The listing builds one solid part. Answer for the finished solid, in the listing's coordinates (mm). A direction names the side the tool comes from. Coordinates: 2 decimals unless noted, no trailing zeros. Order: outer loops, then holes, each group sorted by start corner. A loop starts at its lowest first (then second) coordinate and runs counter-clockwise, first axis right, second up. Notation, with made-up numbers: (89, 37.25) - (125, 37.25) arc R9 ccw to (125, 44.25) - close; hole circle Ø7 at (76, -5.75). An arc over 180 degrees is marked (long way). Use one line per item in the form item = value. Start each with the question number.
Item 1: Consider line 1 along Y through (x, z) = (142, 17.75); line 2 along X through (y, z) = (-28.5, 3); line 3 along X through (y, z) = (-70.5, 5.5). Determine where each line is inside the solid, lowest interval first. Write a range as [from, to].
Item 2: Section B-B, the plane x = 187.5 is taken. Write down the section's boundary in (y, z), and give its area (3 significant figures).
Item 3: The mould has two halves that part along Y. Classify faces 1 (the flat face through (355, 27, 8.89)), 2 (the flat face through (354, -2, 0)): released by +Y, released by -Y, zero draft, split by the parting line, or undercut.
Item 4: Each of these flat-tipped pins is pushed along its axis until it touches: pin 1 Ø1.9 at (y, z) = (31.5, 4) entering from -X; pin 2 Ø2 at (y, z) = (74.5, 12) entering from -X; pin 3 Ø23 at (x, y) = (342.5, -32.5) entering from +Z; pin 4 Ø1.9 at (y, z) = (28.5, 2) entering from +X. Where does it stop, or does it pass through?
Item 5: A tool of negligible diameter and unlimited length cuts with its end or side. For faces 3 (the flat face through (355, 88, 8.89)), 4 (the flat face through (354, -2, 19.05)), from which of +Z, -Z, +X, -X, +Y, -Y can it reach the whole face along a straight path? Write none if from no direction.
from build123d import *

# Parameters (mm, degrees)
F0_W     = 1282.7
F0_H     = 304.8
F1_DEPTH = 19.05
F2_SIZE  = 19.04999
F3_W     = 1092.2
F3_H     = 21.082
F4_DEPTH = 10.16
F6_DEPTH = 6.35


# Not quite as in the source:
# - a fillet or chamfer is up to 0.001 mm smaller than in the source, because OpenCascade refuses the exact size


with BuildPart() as f1:
    # F0 (on Top) → F1 (new body)
    with BuildSketch(Plane.XY):
        with Locations((362.7905342946, -3.9232242852)):
            Rectangle(F0_W, F0_H)
    extrude(amount=F1_DEPTH)

    # F2 (size 19.05 in the source; OpenCascade refuses exactly that, so slightly less here)
    f2_edges = [f1.edges().sort_by_distance(p)[0] for p in [
        (1004.140534, -3.923224, 19.05),
        (-278.559466, -3.923224, 19.05),
    ]]
    chamfer(f2_edges, length=F2_SIZE)

    # F3 (on face) → F4 (cut)
    with BuildSketch(Plane.XY.offset(19.05)):
        with Locations((362.7905342946, 87.5167757148)):
            Rectangle(F3_W, F3_H)
        with Locations((362.7905342946, 26.5567757148)):
            Rectangle(F3_W, F3_H)
        with Locations((362.7905342946, -34.4032242852)):
            Rectangle(F3_W, F3_H)
        with Locations((362.7905342946, -95.3632242852)):
            Rectangle(F3_W, F3_H)
    extrude(amount=-F4_DEPTH, mode=Mode.SUBTRACT)

    # F5 (on face) → F6 (cut)
    with BuildSketch(Plane(origin=(0, 0, 0), x_dir=(1, 0, 0), z_dir=(0, 0, -1))):
        Polygon((899.3655342946, 105.9042242852), (899.3655342946, -98.0577757148), (908.8905342946, -98.0577757148), (908.8905342946, -0.8392757148), (1004.1405342946, -0.8392757148), (1004.1405342946, 8.6857242852), (908.8905342946, 8.6857242852), (908.8905342946, 105.9042242852), align=None)
        Polygon((-278.5594657054, 8.6857242852), (-278.5594657054, -0.8392757148), (-183.3094657054, -0.8392757148), (-183.3094657054, -98.0577757148), (-173.7844657054, -98.0577757148), (-173.7844657054, 105.9042242852), (-183.3094657054, 105.9042242852), (-183.3094657054, 8.6857242852), align=None)
    extrude(amount=-F6_DEPTH, mode=Mode.SUBTRACT)


solid = f1.part
Response:
q1.line_1 = [-156.32, -105.9], [-84.82, -44.94], [-23.86, 16.02], [37.1, 76.98], [98.06, 148.48]
q1.line_2 = [-275.56, -183.31], [-173.78, 899.37], [908.89, 1001.14]
q1.line_3 = [-273.06, -183.31], [-173.78, 899.37], [908.89, 998.64]
q2.outline = (-156.32, 0) - (148.48, 0) - (148.48, 19.05) - (98.06, 19.05) - (98.06, 8.89) - (76.98, 8.89) - (76.98, 19.05) - (37.1, 19.05) - (37.1, 8.89) - (16.02, 8.89) - (16.02, 19.05) - (-23.86, 19.05) - (-23.86, 8.89) - (-44.94, 8.89) - (-44.94, 19.05) - (-84.82, 19.05) - (-84.82, 8.89) - (-105.9, 8.89) - (-105.9, 19.05) - (-156.32, 19.05) - close
q2.area = 4,950 mm2
q3.face_1 = undercut
q3.face_2 = zero draft
q4.pin_1 = -275.51
q4.pin_2 = -267.56
q4.pin_3 = 19.05
q4.pin_4 = 1003.09
q5.face_3 = +Z
q5.face_4 = +Z, +X, -X, +Y, -Y
